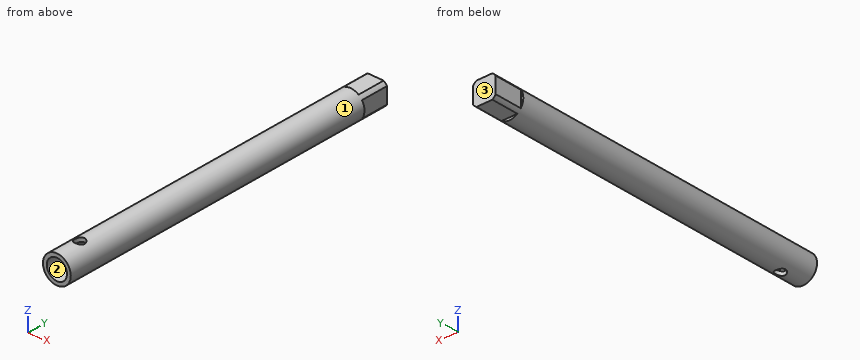
```python
from build123d import *

# Parameters (mm, degrees)
F0_R     = 5.5
F1_DEPTH = 140
F2_R     = 4
F3_DEPTH = 20
F5_DEPTH = 11
F6_R     = 2
F7_DEPTH = 12.5


with BuildPart() as f1:
    # F0 (on Front) → F1 (new body)
    with BuildSketch(Plane.XZ):
        Circle(F0_R)
    extrude(amount=F1_DEPTH)

    # F2 (on face) → F3 (cut)
    with BuildSketch(Plane.XZ.offset(140)):
        Circle(F2_R)
    extrude(amount=-F3_DEPTH, mode=Mode.SUBTRACT)

    # F4 (on face) → F5 (cut)
    with BuildSketch(Plane(origin=(0, 0, 0), x_dir=(-1, 0, 0), z_dir=(0, 1, 0))):
        with BuildLine():
            Line((4.5, 3.1622776602), (4.5, -3.1622776602))
            ThreePointArc((4.5, -3.1622776602), (5.2440442409, -1.6583123952), (5.5, 0))
            ThreePointArc((5.5, 0), (5.2440442409, 1.6583123952), (4.5, 3.1622776602))
        make_face()
        with BuildLine():
            ThreePointArc((3.1622776602, 4.5), (0, 5.5), (-3.1622776602, 4.5))
            Line((-3.1622776602, 4.5), (3.1622776602, 4.5))
        make_face()
        with BuildLine():
            ThreePointArc((-4.5, 3.1622776602), (-5.5, 0), (-4.5, -3.1622776602))
            Line((-4.5, -3.1622776602), (-4.5, 3.1622776602))
        make_face()
        with BuildLine():
            Line((3.1622776602, -4.5), (-3.1622776602, -4.5))
            ThreePointArc((-3.1622776602, -4.5), (0, -5.5), (3.1622776602, -4.5))
        make_face()
    extrude(amount=-F5_DEPTH, mode=Mode.SUBTRACT)

    # F6 (on Top) → F7 (cut, symmetric)
    with BuildSketch(Plane.XY):
        with Locations((0, -130)):
            Circle(F6_R)
    extrude(amount=F7_DEPTH, both=True, mode=Mode.SUBTRACT)


solid = f1.part
```
Design review of the part built by this model. Coordinates are the model's own, in mm. Face numbers are marked on the shaded views. Round coordinates to 2 decimals unless told otherwise and drop trailing zeros. Write each loop counter-clockwise with the first axis right and the second up, starting at its lowest first coordinate (ties: lowest second). Pieces come first, ordered by that corner, then holes.
Item 1: We need section B-B on z = 0. Write out the cut boundary in (x, y).
Item 2: We need section A-A on x = 0. Write out the cut boundary in (y, z), and give its area (3 significant figures).
Item 3: For probe 1 along Y at (x, z) = (0, 4.05); probe 2 along Y at (x, z) = (0, 4.7); probe 3 along Y at (x, z) = (0.75, 3.5), list the stretches that pass through material, from the lowest coordinate up.
Item 4: Clearance check with flat-ended pins moving along their axes: pin 1 Ø3 at (y, z) = (-7.5, 1) entering from +X; pin 2 Ø3 at (x, y) = (-4.5, -85.5) entering from +Z; pin 3 Ø5 at (y, z) = (-6, 1) entering from -X; pin 4 Ø3 at (x, y) = (0, -130) entering from +Z. State where each tip first meets the part, or that it passes through.
Item 5: We need section D-D on y = -102. Write out the cut boundary in (x, z), and give its area (3 significant figures).
Item 6: The part is to be moulded in two halves that separate along X. For the marked faces 1, 2 and 3, say which applies: +X half, -X half, draft (parallel to the pull), parting line (faces both ways), or undercut.
Item 7: We need section C-C on y = -130. Write out the cut boundary in (x, z).
Returned:
1. outline: (-5.5, -140) - (-4, -140) - (-4, -120) - (4, -120) - (4, -140) - (5.5, -140) - (5.5, -11) - (4.5, -11) - (4.5, 0) - (-4.5, 0) - (-4.5, -11) - (-5.5, -11) - close
2. outline: (-140, -5.5) - (-132, -5.5) - (-132, -4) - (-140, -4) - close; (-140, 4) - (-132, 4) - (-132, 5.5) - (-140, 5.5) - close; (-128, -5.5) - (-11, -5.5) - (-11, -4.5) - (0, -4.5) - (0, 4.5) - (-11, 4.5) - (-11, 5.5) - (-128, 5.5) - (-128, 4) - (-120, 4) - (-120, -4) - (-128, -4) - close
2. area: 1,350 mm2
3. probe 1: y = -140 to -132, -128 to 0
3. probe 2: y = -140 to -132, -128 to -11
3. probe 3: y = -120 to 0
4. pin 1: stops at x = 4.5
4. pin 2: stops at z = 4.61
4. pin 3: stops at x = -4.5
4. pin 4: passes through
5. outline: circle Ø11 at (0, 0)
5. area: 95.0 mm2
6. face 1: parting line
6. face 2: undercut
6. face 3: draft
7. outline: (-2, -5.12) - (-2, -3.46) arc R4 cw to (-2, 3.46) - (-2, 5.12) arc R5.5 ccw to start; (2, -5.12) arc R5.5 ccw to (2, 5.12) - (2, 3.46) arc R4 cw to (2, -3.46) - close
